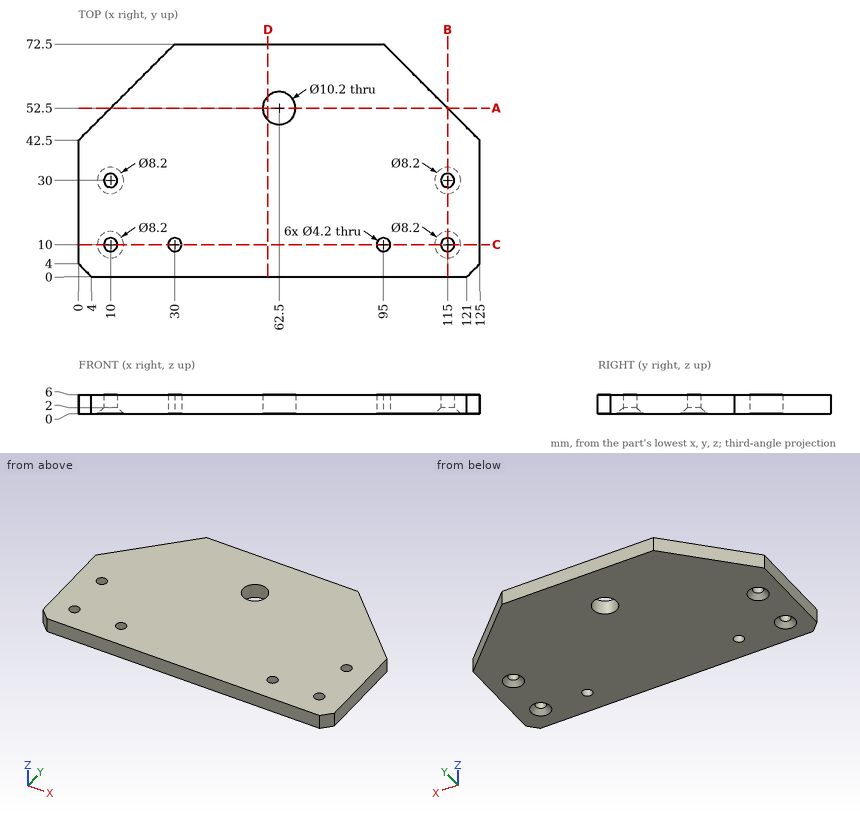
Can you work these out from the drawing? Everything is in mm from the part's minimum corner. Round coordinates to 2 decimals unless told otherwise and drop trailing zeros. Loops run counter-clockwise (first coordinate to the right, second up) from the corner with the lowest first, then second, coordinate; pieces in that order, holes last.
1. If we section it at D-D on x = 59: Write out the boundary of the cut face in (y, z), plus the area to 3 significant figures.
Answer list:
outline: (0, 0) - (48.79, 0) - (48.79, 6) - (0, 6) - close; (56.21, 0) - (72.5, 0) - (72.5, 6) - (56.21, 6) - close
area: 390 mm2
2. For P1, Ø2, axis at y = 48.5, z = 4.5, coming from the -X side; P2, Ø1.5, axis at y = 58.5, z = 5, coming from the +X side; P3, Ø4, axis at x = 10, y = 30, coming from the -Z side, each with a flat end and sliding along its axis, tell me the tip position at first contact or that it passes through.
Answer list:
P1: stops at x = 5
P2: stops at x = 109.75
P3: passes through
3. If I drill on line 1 along Y through (x, z) = (10, 4.45); line 2 along Y through (x, z) = (95, 2.25); line 3 along X through (y, z) = (29.5, 1.25), over which ranges is the centre line in solid material (lowest first)?
Answer list:
line 1: y = 0 to 7.9, 12.1 to 27.9, 32.1 to 52.5
line 2: y = 0 to 7.9, 12.1 to 72.5
line 3: x = 0 to 7.19, 12.81 to 112.19, 117.81 to 125
4. If we section it at A-A on y = 52.5: Write out the boundary of the cut face in (x, z).
Answer list:
outline: (10, 0) - (57.4, 0) - (57.4, 6) - (10, 6) - close; (67.6, 0) - (115, 0) - (115, 6) - (67.6, 6) - close
5. If we section it at B-B on x = 115: Write out the boundary of the cut face in (y, z), plus the area to 3 significant figures.
Answer list:
outline: (0, 0) - (5.9, 0) - (7.9, 2) - (7.9, 6) - (0, 6) - close; (12.1, 2) - (14.1, 0) - (25.9, 0) - (27.9, 2) - (27.9, 6) - (12.1, 6) - close; (32.1, 2) - (34.1, 0) - (52.5, 0) - (52.5, 6) - (32.1, 6) - close
area: 257 mm2
6. If we section it at C-C on y = 10: Write out the boundary of the cut face in (x, z).
Answer list:
outline: (0, 0) - (5.9, 0) - (7.9, 2) - (7.9, 6) - (0, 6) - close; (12.1, 2) - (14.1, 0) - (27.9, 0) - (27.9, 6) - (12.1, 6) - close; (32.1, 0) - (92.9, 0) - (92.9, 6) - (32.1, 6) - close; (97.1, 0) - (110.9, 0) - (112.9, 2) - (112.9, 6) - (97.1, 6) - close; (117.1, 2) - (119.1, 0) - (125, 0) - (125, 6) - (117.1, 6) - close
